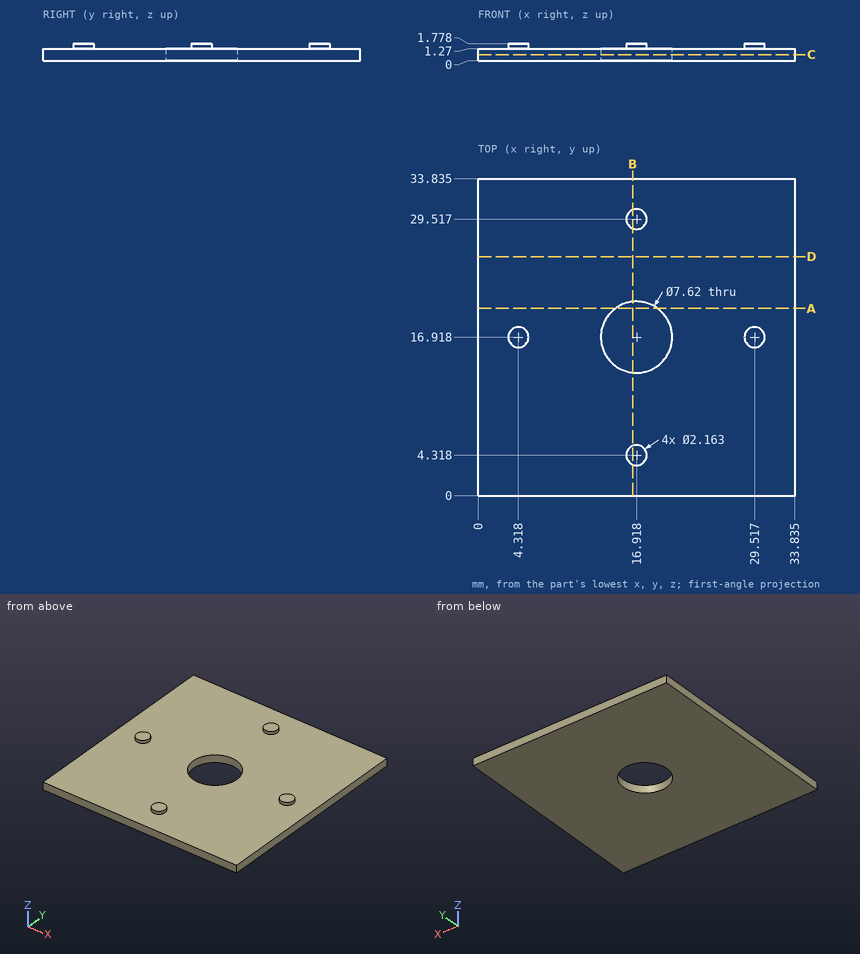
Drawing for the job (mm, zero at the part's lowest x, y, z). Round coordinates to 2 decimals unless told otherwise and drop trailing zeros. Write each loop counter-clockwise with the first axis right and the second up, starting at its lowest first coordinate (ties: lowest second). Pieces come first, ordered by that corner, then holes. Notation, with made-up numbers: (-20.5, 21.25) - (7.5, 21.25) arc R24 ccw to (7.5, 37.25) - close; hole circle Ø4 at (-33.5, 33.25). An arc over 180 degrees is marked (long way). Write item = value, one per line. Start each with the question number.
Q1. Band-saw the part on B-B (x = 16.5). Give the cut face in (y, z) (1 decimal).
Q2. Probe L1, parallel to Z at x = 7, y = 5; L2, parallel to Y at x = 16, z = 1.65 (1 decimal). List the from-to ranges inside material, lowest first. Write a range as from..to.
Q3. Band-saw the part on D-D (y = 25.5). Give the cut face in (x, z) (1 decimal).
Q4. Band-saw the part on C-C (z = 0.65). Give the cut face in (x, y) (1 decimal), then the cut area to 3 significant figures.
Q5. Drop flat-ended pins along their axis: pin 1 (17 mm diameter, centred on x = 20, y = 11.5, fed in from +Z); pin 2 (1 mm diameter, centred on x = 19.5, y = 20.5, fed in from +Z). Give the stop position or say it passes through.
Q6. Band-saw the part on A-A (y = 20). Give the cut face in (x, z) (1 decimal).
Answers below:
q1.outline = (0, 0) - (13.1, 0) - (13.1, 1.3) - (5.3, 1.3) - (5.3, 1.8) - (3.3, 1.8) - (3.3, 1.3) - (0, 1.3) - close; (20.7, 0) - (33.8, 0) - (33.8, 1.3) - (30.5, 1.3) - (30.5, 1.8) - (28.5, 1.8) - (28.5, 1.3) - (20.7, 1.3) - close
q2.L1 = 0..1.27
q2.L2 = 3.7..4.9, 28.9..30.1
q3.outline = (0, 0) - (33.8, 0) - (33.8, 1.3) - (0, 1.3) - close
q4.outline = (0, 0) - (33.8, 0) - (33.8, 33.8) - (0, 33.8) - close; hole circle Ø7.6 at (16.9, 16.9)
q4.area = 1,100 mm2
q5.pin_1 = 1.78
q5.pin_2 = 1.27
q6.outline = (0, 0) - (14.7, 0) - (14.7, 1.3) - (0, 1.3) - close; (19.2, 0) - (33.8, 0) - (33.8, 1.3) - (19.2, 1.3) - close
